Input: part model. Units: mm. Frame: model coordinates. Face numbers are marked on the shaded views. A direction names the side the tool comes from. Round coordinates to 2 decimals unless told otherwise and drop trailing zeros. Write each loop counter-clockwise with the first axis right and the second up, starting at its lowest first coordinate (ties: lowest second). Pieces come first, ordered by that corner, then holes. Notation, with made-up numbers: (-31, 22.5) -> (-3, 22.5) arc R14 ccw to (-3, 36.5) -> close; hole circle Ø9 at (54.25, -15.75). An arc over 180 degrees is marked (long way). Use CSV: the item, a comma, the result in double quotes.
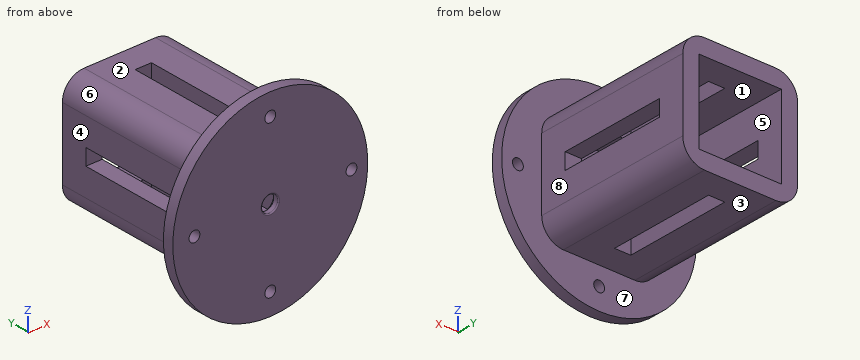
```python
from build123d import *

# Parameters (mm, degrees)
SKETCH1_W           = 21.2
SKETCH1_H           = 21.2
SKETCH1_W_2         = 15.2
SKETCH1_H_2         = 15.2
BOSS_EXTRUDE1_DEPTH = 30
FILLET1_R           = 4
SKETCH3_R           = 18
BOSS_EXTRUDE2_DEPTH = 2
CUT_EXTRUDE2_REACH  = 41.345
SKETCH4_R           = 1.5
SKETCH5_W           = 3
SKETCH5_H           = 20
CUT_EXTRUDE3_DEPTH  = 46.188051518
SKETCH6_W           = 3
SKETCH6_H           = 20
CUT_EXTRUDE4_DEPTH  = 46.188051518
SKETCH7_R           = 1
CUT_EXTRUDE5_DEPTH  = 2
FILLET4_SIZE        = 1
FILLET5_R           = 0.2


with BuildPart() as part:
    # Sketch1 → Boss-Extrude1 (new body)
    with BuildSketch(Plane(origin=(0, 0, 0), x_dir=(1, 0, 0), z_dir=(0, 1, 0))):
        Rectangle(SKETCH1_W, SKETCH1_H)
        Rectangle(SKETCH1_W_2, SKETCH1_H_2, mode=Mode.SUBTRACT)
    extrude(amount=BOSS_EXTRUDE1_DEPTH)

    # Fillet1
    fillet1_edges = [part.edges().sort_by_distance(p)[0] for p in [
        (10.6, 15, 10.6),
        (-10.6, 15, 10.6),
        (-10.6, 15, -10.6),
        (10.6, 15, -10.6),
    ]]
    fillet(fillet1_edges, radius=FILLET1_R)

    # Sketch3 → Boss-Extrude2 (add)
    with BuildSketch(Plane.XZ):
        with Locations(Location((0, 0, 0), (0, 0, 270))):
            Circle(SKETCH3_R)
    extrude(amount=BOSS_EXTRUDE2_DEPTH)

    # Sketch4 → Cut-Extrude2 (cut, up to next)
    with BuildSketch(Plane(origin=(0, 0, 0), x_dir=(1, 0, 0), z_dir=(0, 1, 0)), mode=Mode.PRIVATE) as cut_extrude2_sk1:
        with Locations(Location((0, 0, 0), (0, 0, 270))):
            Circle(SKETCH4_R)
    cut_extrude2_tool1 = extrude(cut_extrude2_sk1.sketch, amount=-CUT_EXTRUDE2_REACH, mode=Mode.PRIVATE) & part.part
    add(cut_extrude2_tool1.solids().sort_by_distance((0, 0, 0))[0], mode=Mode.SUBTRACT)

    # Sketch5 → Cut-Extrude3 (cut, through all)
    with BuildSketch(Plane(origin=(0, 0, -10.6), x_dir=(-1, 0, 0), z_dir=(0, 0, -1))):
        with Locations((0, 15)):
            Rectangle(SKETCH5_W, SKETCH5_H)
    extrude(amount=-CUT_EXTRUDE3_DEPTH, mode=Mode.SUBTRACT)

    # Sketch6 → Cut-Extrude4 (cut, through all)
    with BuildSketch(Plane(origin=(10.6, 0, 0), x_dir=(0, 0, -1), z_dir=(1, 0, 0))):
        with Locations((0, 15)):
            Rectangle(SKETCH6_W, SKETCH6_H)
    extrude(amount=-CUT_EXTRUDE4_DEPTH, mode=Mode.SUBTRACT)

    # Sketch7 → Cut-Extrude5 (cut)
    with BuildSketch(Plane(origin=(0, -2, 0), x_dir=(-1, 0, 0), z_dir=(0, -1, 0))):
        with Locations(Location((14, 0, 0), (0, 0, 90))):
            Circle(SKETCH7_R)
        with Locations(Location((-15, 0, 0), (0, 0, 270))):
            Circle(SKETCH7_R)
        with Locations(Location((0, 14, 0), (0, 0, 90))):
            Circle(SKETCH7_R)
        with Locations(Location((0, -14, 0), (0, 0, 270))):
            Circle(SKETCH7_R)
    extrude(amount=-CUT_EXTRUDE5_DEPTH, mode=Mode.SUBTRACT)

    # Fillet4
    # a fillet whose section is not a circle: 1 mm, written as the material it takes off along each edge
    with BuildSketch(Plane(origin=(0, 0, 0), x_dir=(0, 0, 1), z_dir=(-1, 0, 0))) as fillet4_piece_1:
        with BuildLine():
            Bezier((1.5, -FILLET4_SIZE), (1.5, 0), (1.5 + FILLET4_SIZE, 0), weights=[1, 0.070710678, 1])
            Line((1.5 + FILLET4_SIZE, 0), (1.5, 0))
            Line((1.5, 0), (1.5, -FILLET4_SIZE))
        make_face()
    revolve(axis=Axis((0, 0, 0), (0, 1, 0)), mode=Mode.SUBTRACT)

    # Fillet5
    fillet5_edges = [part.edges().sort_by_distance(p)[0] for p in [
        (0, -2, -1.5),
    ]]
    fillet(fillet5_edges, radius=FILLET5_R)


solid = part.part
```
Item 1: Section query D-D on z = 0. Give the number of separate pieces and of enclosed holes in the cut face, plus the area to 3 significant figures.
Worked answers:
separate pieces,"6"
enclosed holes,"0"
area,"117 mm²"
Item 2: First-contact query: pin 1 Ø3.5 at (y, z) = (15.5, 8.5) entering from -X; pin 2 Ø1.5 at (y, z) = (17.5, 5.5) entering from +X; pin 3 Ø16.5 at (x, z) = (0, 1) entering from +Y; pin 4 Ø2.5 at (x, z) = (-14, 0) entering from +Y. Flat tips, straight axial feed; report the tip coordinate or a pass-through.
Worked answers:
pin 1,"stops at x = -10.6"
pin 2,"stops at x = 10.6"
pin 3,"stops at y = 30"
pin 4,"stops at y = 0"
Item 3: Section query C-C on z = 14.5. Return the cut outline in (x, y), plus the area to 3 significant figures.
Worked answers:
outline,"(-10.67, -2) -> (-0.87, -2) -> (-0.87, 0) -> (-10.67, 0) -> close; (0.87, -2) -> (10.67, -2) -> (10.67, 0) -> (0.87, 0) -> close"
area,"39.2 mm²"
Item 4: Line query: line 1 (X direction, y = -0.75, z = 0); line 2 (X direction, y = -1.2, z = 0); line 3 (X direction, y = 24, z = 2.5). Output: solid intervals per line, ascending.
Worked answers:
line 1,"x = -18 to -15, -13 to -1.7, 1.7 to 14, 16 to 18"
line 2,"x = -18 to -15, -13 to -1.5, 1.5 to 14, 16 to 18"
line 3,"x = -10.6 to -7.6, 7.6 to 10.6"
Item 5: Set-up query: the marked faces 1, 2, 3 and 4. Return all of +Z, -Z, +X, -X, +Y, -Y with unobstructed straight access to the full face (end or side cutting, diameter ignored); none if empty.
Worked answers:
face 1,"+Y"
face 2,"+Z, +X, -X, +Y"
face 3,"-Z, +X, -X, +Y"
face 4,"+Z, -Z, -X, +Y"
Item 6: Section query A-A on y = 23. Return the cut outline in (x, z), plus the area to 3 significant figures.
Worked answers:
outline,"(-10.6, -6.6) arc R4 ccw to (-6.6, -10.6) -> (-1.5, -10.6) -> (-1.5, -7.6) -> (-7.6, -7.6) -> (-7.6, -1.5) -> (-10.6, -1.5) -> close; (-10.6, 1.5) -> (-7.6, 1.5) -> (-7.6, 7.6) -> (-1.5, 7.6) -> (-1.5, 10.6) -> (-6.6, 10.6) arc R4 ccw to (-10.6, 6.6) -> close; (1.5, -10.6) -> (6.6, -10.6) arc R4 ccw to (10.6, -6.6) -> (10.6, -1.5) -> (7.6, -1.5) -> (7.6, -7.6) -> (1.5, -7.6) -> close; (1.5, 7.6) -> (7.6, 7.6) -> (7.6, 1.5) -> (10.6, 1.5) -> (10.6, 6.6) arc R4 ccw to (6.6, 10.6) -> (1.5, 10.6) -> close"
area,"169 mm²"
Item 7: Pull-direction query (X, two-part tool) for the marked faces 5, 6, 7 and 8; classes: +X half, -X half, draft (parallel to the pull), parting line (faces both ways), or undercut.
Worked answers:
face 5,"undercut"
face 6,"-X half"
face 7,"draft"
face 8,"+X half"
Item 8: Section query B-B on x = -14. Return the cut outline in (y, z), plus the area to 3 significant figures.
Worked answers:
outline,"(-2, -11.31) -> (0, -11.31) -> (0, -1) -> (-2, -1) -> close; (-2, 1) -> (0, 1) -> (0, 11.31) -> (-2, 11.31) -> close"
area,"41.3 mm²"
